Can you work these out from the model? Positions are in its coordinate system, mm. A direction names the side the tool comes from. Coordinates: 2 decimals unless noted, no trailing zeros. Write each loop counter-clockwise with the first axis right and the second up, starting at its lowest first coordinate (ties: lowest second). Pieces come first, ordered by that corner, then holes. Notation, with made-up numbers: (28.25, 81.5) - (87.25, 81.5) arc R21 cw to (87.25, 94.5) - close; hole circle Ø8 at (71, 4.5). An arc over 180 degrees is marked (long way). One line per question, with ' | ' between items. Start each with the question number.
from build123d import *

# Parameters (mm, degrees)
SKETCH2_W            = 83
SKETCH2_H            = 100
BOSS_EXTRUDE1_DEPTH  = 1.75
SKETCH3_W            = 18
SKETCH3_H            = 18
CUT_EXTRUDE5_DEPTH   = 0.2
LPATTERN1_COUNT      = 4
LPATTERN1_PITCH      = 20
LPATTERN1_COUNT_DIR2 = 5
LPATTERN1_PITCH_DIR2 = 20


with BuildPart() as part:
    # Sketch2 → Boss-Extrude1 (new body)
    with BuildSketch(Plane(origin=(0, 0, 0), x_dir=(1, 0, 0), z_dir=(0, 1, 0))):
        Rectangle(SKETCH2_W, SKETCH2_H)
    extrude(amount=BOSS_EXTRUDE1_DEPTH)

    # Sketch3 → Cut-Extrude5 (cut)
    with BuildSketch(Plane(origin=(0, 0, 0), x_dir=(1, 0, 0), z_dir=(0, 1, 0))):
        with Locations((-30.5, 39)):
            Rectangle(SKETCH3_W, SKETCH3_H)
    cut_extrude5 = extrude(amount=CUT_EXTRUDE5_DEPTH, mode=Mode.SUBTRACT)

    # LPattern1: Cut-Extrude5 4 × 5
    with Locations(*[(i * LPATTERN1_PITCH, 0, j * LPATTERN1_PITCH_DIR2) for i in range(LPATTERN1_COUNT) for j in range(LPATTERN1_COUNT_DIR2) if (i, j) != (0, 0)]):
        add(cut_extrude5, mode=Mode.SUBTRACT)


solid = part.part
(1) Which directions (+Z, -Z, +X, -X, +Y, -Y) give clear straight access to the entire face, cutting with the end or side of a thin tool? Please do faces 3 (the face through (-31, 0.2, 1)), 4 (the face through (-11, 0.2, 41)).
(2) I'm going to push a flat-ended pin straight in: pin 1 (9 mm diameter, centred on x = -8.5, z = 3.5, fed in from -Y). Where does the tip first touch, or does it pass through?
(3) If we mould it in two halves opening along X, with no side actions, what happens to faces 1 (the face through (0, 0, -8)), 2 (the face through (9, 0.2, -19))? For each: +X half, -X half, draft (parallel to the pull), parting line (faces both ways), or undercut.
(4) If I drill on probe 1 along X at (y, z) = (0.15, -32.5); probe 2 along Y at (x, z) = (-4.5, -25), over which ranges is the centre line in solid material (lowest first)?
(5) If we section it at B-B on z = -26: List the corners of the cut face in (x, y) for me.
(6) If we section it at A-A on x = 28: List the corners of the cut face in (y, z) for me, plus the area to 3 significant figures.
Values:
1) face 3: -Y | face 4: +Z, -Y
2) pin 1: y = 0.2
3) face 1: draft | face 2: undercut
4) probe 1: -41.5 to -39.5, -21.5 to -19.5, -1.5 to 0.5, 18.5 to 20.5, 38.5 to 41.5 | probe 2: 0.2 to 1.75
5) outline: (-41.5, 0) - (-39.5, 0) - (-39.5, 0.2) - (-21.5, 0.2) - (-21.5, 0) - (-19.5, 0) - (-19.5, 0.2) - (-1.5, 0.2) - (-1.5, 0) - (0.5, 0) - (0.5, 0.2) - (18.5, 0.2) - (18.5, 0) - (20.5, 0) - (20.5, 0.2) - (38.5, 0.2) - (38.5, 0) - (41.5, 0) - (41.5, 1.75) - (-41.5, 1.75) - close
6) outline: (0, -50) - (1.75, -50) - (1.75, 50) - (0.2, 50) - (0.2, 32) - (0, 32) - (0, 30) - (0.2, 30) - (0.2, 12) - (0, 12) - (0, 10) - (0.2, 10) - (0.2, -8) - (0, -8) - (0, -10) - (0.2, -10) - (0.2, -28) - (0, -28) - (0, -30) - (0.2, -30) - (0.2, -48) - (0, -48) - close | area: 157 mm2
